```python
from build123d import *

# Parameters (mm, degrees)
EXTRUDE_1_DEPTH     = 7
SKETCH_2_R          = 2.5
CUT_EXTRUDE_1_DEPTH = 10
SKETCH_3_W          = 34
SKETCH_3_H          = 36
EXTRUDE_2_DEPTH     = 38
SKETCH_6_R          = 14
CUT_EXTRUDE_2_DEPTH = 40
SKETCH_8_W          = 4
SKETCH_8_H          = 36
CUT_EXTRUDE_3_DEPTH = 10
FILLET_1_R          = 10


with BuildPart() as part:
    # 草圖1 → 填料-伸長1 (new body)
    with BuildSketch(Plane.XY):
        with BuildLine():
            Line((35.5, -18), (-35.5, -18))
            ThreePointArc((-35.5, -18), (-42.571067812, -15.071067812), (-45.5, -8))
            Line((-45.5, -8), (-45.5, 8))
            ThreePointArc((-45.5, 8), (-42.571067812, 15.071067812), (-35.5, 18))
            Line((-35.5, 18), (35.5, 18))
            ThreePointArc((35.5, 18), (42.571067812, 15.071067812), (45.5, 8))
            Line((45.5, 8), (45.5, -8))
            ThreePointArc((45.5, -8), (42.571067812, -15.071067812), (35.5, -18))
        make_face()
    extrude(amount=EXTRUDE_1_DEPTH)

    # 草圖2 → 除料-伸長1 (cut)
    with BuildSketch(Plane.XY.offset(7)):
        with Locations((-35.5, 10)):
            Circle(SKETCH_2_R)
        with Locations((35.5, 10)):
            Circle(SKETCH_2_R)
        with Locations((35.5, -10)):
            Circle(SKETCH_2_R)
        with Locations((-35.5, -10)):
            Circle(SKETCH_2_R)
    extrude(amount=-CUT_EXTRUDE_1_DEPTH, mode=Mode.SUBTRACT)

    # 草圖3 → 填料-伸長2 (add)
    with BuildSketch(Plane.XY.offset(7)):
        Rectangle(SKETCH_3_W, SKETCH_3_H)
    extrude(amount=EXTRUDE_2_DEPTH)

    # 草圖6 → 除料-伸長2 (cut)
    with BuildSketch(Plane(origin=(0, 18, 0), x_dir=(1, 0, 0), z_dir=(0, 1, 0))):
        with Locations(Location((0, -27, 0), (0, 0, 180))):
            Circle(SKETCH_6_R)
    extrude(amount=-CUT_EXTRUDE_2_DEPTH, mode=Mode.SUBTRACT)

    # 草圖8 → 除料-伸長3 (cut)
    with BuildSketch(Plane.XY.offset(45)):
        Rectangle(SKETCH_8_W, SKETCH_8_H)
    extrude(amount=-CUT_EXTRUDE_3_DEPTH, mode=Mode.SUBTRACT)

    # 圓角1
    fillet_1_edges = [part.edges().sort_by_distance(p)[0] for p in [
        (-17, 0, 45),
        (17, 0, 45),
    ]]
    fillet(fillet_1_edges, radius=FILLET_1_R)


solid = part.part
```
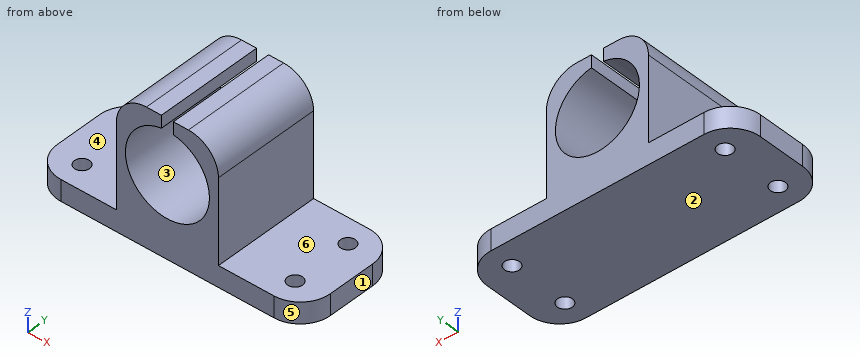
Geometry: final body of the model. Coordinates: model frame, mm. Face numbers are marked on the shaded views. A direction names the side the tool comes from. Round coordinates to 2 decimals unless told otherwise and drop trailing zeros. Order: outer loops, then holes, each group sorted by start corner. A loop starts at its lowest first (then second) coordinate and runs counter-clockwise, first axis right, second up. Notation, with made-up numbers: M 30,-8.75 L 37,-8.75 A22 cw 37,3.25 Z; hole C 17.25,58.5 d8. An arc over 180 degrees is marked long. One line per item, written item: value.
(1) Line query: probe 1 along Y at (x, z) = (35.5, 1.5); probe 2 along X at (y, z) = (-4, 27); probe 3 along Y at (x, z) = (35, 3). Output: solid intervals per line, ascending. Write a range as [from, to].
Result sheet:
probe 1: [-18, -12.5], [-7.5, 7.5], [12.5, 18]
probe 2: [-17, -14], [14, 17]
probe 3: [-18, -12.45], [-7.55, 7.55], [12.45, 18]
(2) Cut plane D-D (x = -3). Return the cut outline in (y, z).
Result sheet:
outline: M -18,0 L 18,0 L 18,13.33 L -18,13.33 Z; M -18,40.67 L 18,40.67 L 18,45 L -18,45 Z
(3) Cut plane A-A (x = 34). Return the cut outline in (y, z), and give its area (3 significant figures).
Result sheet:
outline: M -18,0 L -12,0 L -12,7 L -18,7 Z; M -8,0 L 8,0 L 8,7 L -8,7 Z; M 12,0 L 18,0 L 18,7 L 12,7 Z
area: 196 mm2
(4) Cut plane C-C (y = 6). Return the cut outline in (x, z), and give its area (3 significant figures).
Result sheet:
outline: M -45.5,0 L 45.5,0 L 45.5,7 L 17,7 L 17,35 A10 ccw 7,45 L 2,45 L 2,40.86 A14 cw long -2,40.86 L -2,45 L -7,45 A10 ccw -17,35 L -17,7 L -45.5,7 Z
area: 1,250 mm2
(5) Reachability of the marked faces 4, 5 and 6 from +Z, -Z, +X, -X, +Y, -Y: full face, straight path, thin tool, end or side. Return the list, or none.
Result sheet:
face 4: +Z, -X, +Y, -Y
face 5: +Z, -Z, +X, -Y
face 6: +Z, +X, +Y, -Y
(6) Cut plane B-B (z = 27). Return the cut outline in (x, y), and give its area (3 significant figures).
Result sheet:
outline: M -17,-18 L -14,-18 L -14,18 L -17,18 Z; M 14,-18 L 17,-18 L 17,18 L 14,18 Z
area: 216 mm2
(7) Pin query (flat end, axial travel): P1, Ø3.5, axis at y = -6, z = 42, coming from the -X side; P2, Ø1, axis at y = 7.5, z = 36, coming from the +X side; P3, Ø6, axis at x = 35.5, y = -10, coming from the +Z side. Return the tip coordinate at first contact, or that it passes through.
Result sheet:
P1: x = -15.51
P2: x = 16.99
P3: z = 7
(8) Pull-direction query (Z, two-part tool) for the marked faces 1, 2 and 3; classes: pulls with the +Z half, pulls with the -Z half, needs draft (parallel to the pull), parting line crosses it, or undercut.
Result sheet:
face 1: needs draft
face 2: pulls with the -Z half
face 3: undercut
